Geometry: final body of the model. Coordinates: model frame, mm. A direction names the side the tool comes from. Round coordinates to 2 decimals unless told otherwise and drop trailing zeros. Write each loop counter-clockwise with the first axis right and the second up, starting at its lowest first coordinate (ties: lowest second). Pieces come first, ordered by that corner, then holes. Notation, with made-up numbers: (62.25, 68) -> (120.25, 68) arc R18 ccw to (120.25, 73) -> close; hole circle Ø11 at (41.5, -3.75). An arc over 180 degrees is marked (long way). Use one line per item in the form item = value. Start each with the question number.
1. Reachability of faces 1 (the face through (-38.108, -48, 2)), 2 (the face through (-11, -15.678, 2)), 3 (the face through (-9.695, -6.895, 1.972)) from +Z, -Z, +X, -X, +Y, -Y: full face, straight path, thin tool, end or side. Return the list, or none.
2. Line query: L1, parallel to X at y = -7.5, z = 0.7; L2, parallel to Y at x = -51, z = 1.45; L3, parallel to X at y = -4, z = 2.6. Output: solid intervals per line, ascending.
3. Cut plane C-C, the plane y = -45.5. Return the cut outline in (x, z), plus the area to 3 significant figures.
4. Pin query (flat end, axial travel): pin 1 Ø1.2 at (y, z) = (-49.5, 2.5) entering from -X; pin 2 Ø2 at (x, z) = (-10, 2.5) entering from -Y. Return the tip coordinate at first contact, or that it passes through.
5. Cut plane B-B, the plane x = -85. Return the cut outline in (y, z).
6. Draft query along Y for faces 4 (the face through (-96.2, -5.08, 1.97)), 5 (the face through (-37, -20, 4)), 6 (the face through (-27.033, -73.992, 1.972)), 7 (the face through (-39.612, -17.104, 1.972)). Return one class per face: pulls with the +Y half, pulls with the -Y half, needs draft (parallel to the pull), parting line crosses it, or undercut.
7. Cut plane A-A, the plane z = 1.8. Return the cut outline in (x, y), plus the area to 3 significant figures.
```python
from build123d import *

# Parameters (mm, degrees)
SKETCH_1_R      = 2
EXTRUDE_1_DEPTH = 4


with BuildPart() as part:
    # 草图1 → 凸台-拉伸1 (new body)
    with BuildSketch(Plane.XY):
        with BuildLine():
            Line((-98.108217502, -15.678085124), (-43.108217502, -15.678085124))
            ThreePointArc((-43.108217502, -15.678085124), (-39.572683597, -17.142551218), (-38.108217502, -20.678085124))
            Line((-38.108217502, -20.678085124), (-38.108217502, -75.678085124))
            ThreePointArc((-38.108217502, -75.678085124), (-28.108217502, -85.678085124), (-18.108217502, -75.678085124))
            Line((-18.108217502, -75.678085124), (-18.108217502, -20.678085124))
            ThreePointArc((-18.108217502, -20.678085124), (-16.643751408, -17.142551218), (-13.108217502, -15.678085124))
            Line((-13.108217502, -15.678085124), (-8.108217502, -15.678085124))
            ThreePointArc((-8.108217502, -15.678085124), (1.352773969, -8.916856554), (-1.979819728, 2.223986801))
            ThreePointArc((-1.979819728, 2.223986801), (-4.869446073, 3.782906348), (-8.108217502, 4.321914876))
            Line((-8.108217502, 4.321914876), (-98.108217502, 4.321914876))
            ThreePointArc((-98.108217502, 4.321914876), (-108.108217502, -5.678085124), (-98.108217502, -15.678085124))
        make_face()
        with Locations((-28.108217502, -75.678085124)):
            Circle(SKETCH_1_R, mode=Mode.SUBTRACT)
        with Locations((-98.108217502, -5.678085124)):
            Circle(SKETCH_1_R, mode=Mode.SUBTRACT)
        with Locations((-68.608217502, -5.678085124)):
            Circle(SKETCH_1_R, mode=Mode.SUBTRACT)
        with Locations((-8.108217502, -5.678085124)):
            Circle(SKETCH_1_R, mode=Mode.SUBTRACT)
    extrude(amount=EXTRUDE_1_DEPTH)


solid = part.part
```
Outcome:
q1.face_1 = +Z, -Z, -X, -Y
q1.face_2 = +Z, -Z, +X, -Y
q1.face_3 = +Z, -Z
q2.L1 = -107.94 to -98.93, -97.28 to -69.43, -67.78 to -8.93, -7.28 to 1.72
q2.L2 = -15.68 to 4.32
q2.L3 = -107.97 to -99.2, -97.02 to -69.7, -67.52 to -9.2, -7.02 to 1.75
q3.outline = (-38.11, 0) -> (-18.11, 0) -> (-18.11, 4) -> (-38.11, 4) -> close
q3.area = 80.0 mm^2
q4.pin_1 = -38.11
q4.pin_2 = -15.68
q5.outline = (-15.68, 0) -> (4.32, 0) -> (4.32, 4) -> (-15.68, 4) -> close
q6.face_4 = undercut
q6.face_5 = needs draft
q6.face_6 = undercut
q6.face_7 = pulls with the -Y half
q7.outline = (-98.11, -15.68) -> (-43.11, -15.68) arc R5 cw to (-38.11, -20.68) -> (-38.11, -75.68) arc R10 ccw to (-18.11, -75.68) -> (-18.11, -20.68) arc R5 cw to (-13.11, -15.68) -> (-8.11, -15.68) arc R10 ccw to (-8.11, 4.32) -> (-98.11, 4.32) arc R10 ccw to start; hole circle Ø4 at (-98.11, -5.68); hole circle Ø4 at (-68.61, -5.68); hole circle Ø4 at (-28.11, -75.68); hole circle Ø4 at (-8.11, -5.68)
q7.area = 3,430 mm^2
